Design review of the part built by this model. Coordinates are the model's own, in mm. Face numbers are marked on the shaded views. A direction names the side the tool comes from. Coordinates: 2 decimals unless noted, no trailing zeros. Write each loop counter-clockwise with the first axis right and the second up, starting at its lowest first coordinate (ties: lowest second). Pieces come first, ordered by that corner, then holes. Notation, with made-up numbers: (48, 4.25) -> (69, 4.25) arc R22 ccw to (69, 25.25) -> close; hole circle Ø2 at (25.5, -13.75). An arc over 180 degrees is marked (long way). Write item = value, one per line. Start each with the question number.
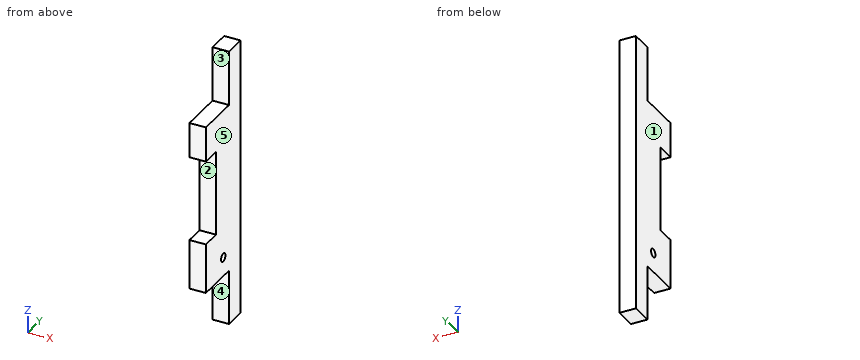
Autodesk Inventor part; units mm, degrees
ref_plane "YZ Plane" through (0, 0, 0) normal (1, 0, 0) x (0, 1, 0)
ref_plane "XZ Plane" through (0, 0, 0) normal (0, 1, 0) x (-1, 0, 0)
ref_plane "XY Plane" through (0, 0, 0) normal (0, 0, 1) x (1, 0, 0)
sketch "Sketch2" plane through (0, 0, 0) normal (1, 0, 0) x (0, 1, 0)
  line L0 (0, 0) -> (0, 95.25)
  line L1 (0, 95.25) -> (50.8, 95.25)
  line L2 (50.8, 95.25) -> (50.8, 158.75)
  line L3 (50.8, 158.75) -> (76.2, 158.75)
  line L4 (76.2, 158.75) -> (76.2, 15.0657)
  line L5 (76.2, 15.0657) -> (76.2, 0)
  line L6 (76.2, 0) -> (0, 0) construction
  line L7 (0, 0) -> (0, -95.25)
  line L8 (0, -95.25) -> (50.8, -95.25)
  line L9 (50.8, -95.25) -> (50.8, -158.75)
  line L10 (50.8, -158.75) -> (76.2, -158.75)
  line L11 (76.2, -158.75) -> (76.2, -15.0657)
  line L12 (76.2, -15.0657) -> (76.2, 0)
  dimension "d5" = 50.8
  dimension "d6" = 25.4
  dimension "d8" = 63.5
  dimension "d9" = 95.25
extrude "Extrusion1" add sketch "Sketch2" along normal mid plane 19.05
sketch "Sketch3" plane through (9.525, 50.8, -95.25) normal (0, 0, -1) x (-1, 0, 0)
  line L0 (19.05, 0) -> (19.05, 25.4)
  line L1 (0, -50.8) -> (19.05, -50.8)
  line L2 (19.05, -50.8) -> (19.05, 0)
  line L3 (19.05, 0) -> (0, 0)
  line L4 (0, 0) -> (0, -50.8)
  point P0 (9.525, -50.8)
extrude "Extrusion2" add sketch "Sketch3" along normal blind 6.35
sketch "Sketch4" plane through (9.525, 76.2, -158.75) normal (0, 0, -1) x (-1, 0, 0)
  line L0 (0, 0) -> (0, -25.4)
  line L1 (19.05, -25.4) -> (19.05, 0)
  line L2 (0, 0) -> (19.05, 0)
  line L3 (19.05, 0) -> (19.05, -25.4)
  line L4 (19.05, -25.4) -> (0, -25.4)
  line L5 (0, -25.4) -> (0, 0)
  point P0 (9.525, -76.2)
extrude "Extrusion3" add sketch "Sketch4" along normal blind 6.35
sketch "Sketch6" plane through (9.525, 0, 0) normal (1, 0, 0) x (0, 0, -1)
  line L0 (-95.25, 50.8) -> (-95.25, 0) construction
  line L1 (-95.25, 38.1) -> (101.6, 38.1) construction
  line L2 (101.6, 50.8) -> (101.6, 0) construction
  line L3 (-158.75, 76.2) -> (165.1, 76.2) construction
  circle A0 centre (79.375, 38.1) radius 4.7625
  line L4 (165.1, 76.2) -> (165.1, 50.8)
  point P0 (0, 0)
  dimension "d28" = 38.1
  dimension "d29" = 85.725
  dimension "d30" = 9.525
extrude "Extrusion5" cut sketch "Sketch6" against normal through all
sketch "Sketch7" plane through (9.525, 0, 0) normal (1, 0, 0) x (0, 0, -1)
  circle A0 centre (79.375, 38.1) radius 4.7625
  line L0 (-95.25, 0) -> (101.6, 0)
  line L1 (-95.25, 0) -> (-95.25, 50.8)
  line L2 (-95.25, 50.8) -> (-158.75, 50.8)
  line L3 (-158.75, 50.8) -> (-158.75, 76.2)
  line L4 (-158.75, 76.2) -> (165.1, 76.2)
  line L5 (165.1, 50.8) -> (165.1, 76.2)
  line L6 (101.6, 50.8) -> (165.1, 50.8)
  line L7 (101.6, 0) -> (101.6, 50.8)
  line L8 (-95.25, 0) -> (101.6, 0)
  line L9 (-54.5452, 0) -> (43.8798, 0)
  line L10 (43.8798, 0) -> (43.8798, 22.225)
  line L11 (43.8798, 22.225) -> (-54.5452, 22.225)
  line L12 (-54.5452, 22.225) -> (-54.5452, 0)
  point P0 (0, 0)
  dimension "d33" = 98.425
  dimension "d34" = 22.225
extrude "Extrusion6" cut sketch "Sketch7" against normal through all contours L12 L11 L10 L0
properties part number "SpanRearAndMiddleSupport" material "Aluminum 6061"
(1) Mouldability with a two-part tool opening along Z and no side actions: class the marked faces 1 and 2 as pulls with the +Z half, pulls with the -Z half, needs draft (parallel to the pull), parting line crosses it, or undercut.
(2) For the marked faces 3, 4 and 5, list the 3-axis set-ups (+Z, -Z, +X, -X, +Y, -Y) from which the entire face can be reached by the end or side of a thin tool; tool diameter is ignored.
(3) Take a section at A-A, the plane y = 15. State the section outline as (x, z) points (3 decimals).
(4) For line 1 (Z direction, x = -6.5, y = 19.5); line 2 (Z direction, x = 8.75, y = 25); line 3 (Y direction, x = 0.5, z = 119.5), list the stretches that pass through material, from the lowest coordinate up.
(5) For pin 1 Ø6 at (x, y) = (0.5, 14) entering from +Z; pin 2 Ø5.5 at (x, z) = (-2.5, 122) entering from -Y; pin 3 Ø5.5 at (x, y) = (4.5, 16) entering from -Z, all flat-tipped, find the tip position at first contact; note any pin that passes through.
(6) Take a section at D-D, the plane z = -144.5. State the section outline as (x, y) points (3 decimals).
Report:
q1.face_1 = needs draft
q1.face_2 = undercut
q2.face_3 = +Z, +X, -X, -Y
q2.face_4 = -Z, +X, -X, -Y
q2.face_5 = +Z, -Z, +X, +Y, -Y
q3.outline = (-9.525, -101.6) -> (9.525, -101.6) -> (9.525, -43.88) -> (-9.525, -43.88) -> close; (-9.525, 54.545) -> (9.525, 54.545) -> (9.525, 95.25) -> (-9.525, 95.25) -> close
q4.line_1 = -101.6 to -43.88, 54.55 to 95.25
q4.line_2 = -101.6 to 95.25
q4.line_3 = 50.8 to 76.2
q5.pin_1 = 95.25
q5.pin_2 = 50.8
q5.pin_3 = -101.6
q6.outline = (-9.525, 50.8) -> (9.525, 50.8) -> (9.525, 76.2) -> (-9.525, 76.2) -> close
